```python
from build123d import *

# Parameters (mm, degrees)
BOSS_EXTRU_1_DEPTH      = 564
ESQUISSE2_W             = 18
ESQUISSE2_H             = 18
ENL_V_MAT_EXTRU_1_DEPTH = 3
ESQUISSE6_R             = 1.4
ENL_V_MAT_EXTRU_5_DEPTH = 3
SKETCH1_R               = 1.6
CUT_EXTRUDE1_DEPTH      = 21


with BuildPart() as part:
    # Esquisse1 → Boss.-Extru.1 (new body)
    with BuildSketch(Plane.XY):
        Polygon((0, 0), (20, 0), (20, 2), (2, 2), (2, 20), (0, 20), align=None)
    extrude(amount=BOSS_EXTRU_1_DEPTH)

    # Esquisse2 → Enlèv. mat.-Extru.1 (cut, through all)
    with BuildSketch(Plane(origin=(2, 0, 0), x_dir=(0, 0, -1), z_dir=(1, 0, 0))):
        with Locations((-555, 11)):
            Rectangle(ESQUISSE2_W, ESQUISSE2_H)
        with Locations((-9, 11)):
            Rectangle(ESQUISSE2_W, ESQUISSE2_H)
    extrude(amount=-ENL_V_MAT_EXTRU_1_DEPTH, mode=Mode.SUBTRACT)

    # Esquisse6 → Enlèv. mat.-Extru.5 (cut, through all)
    with BuildSketch(Plane(origin=(0, 2, 0), x_dir=(1, 0, 0), z_dir=(0, 1, 0))):
        with Locations((6.48, -549.52)):
            Circle(ESQUISSE6_R)
        with Locations((6.48, -14.48)):
            Circle(ESQUISSE6_R)
        with Locations((16.48, -559.52)):
            Circle(ESQUISSE6_R)
        with Locations((16.48, -4.48)):
            Circle(ESQUISSE6_R)
    extrude(amount=-ENL_V_MAT_EXTRU_5_DEPTH, mode=Mode.SUBTRACT)

    # Sketch1 → Cut-Extrude1 (cut, through all)
    with BuildSketch(Plane.ZY):
        with Locations((217, 11)):
            Circle(SKETCH1_R)
        with Locations((347, 11)):
            Circle(SKETCH1_R)
    extrude(amount=-CUT_EXTRUDE1_DEPTH, mode=Mode.SUBTRACT)


solid = part.part
```
Check sheet for the modelled part. Datum: model origin and axes. Units: mm. A direction names the side the tool comes from. Round coordinates to 2 decimals unless told otherwise and drop trailing zeros. Order: outer loops, then holes, each group sorted by start corner. A loop starts at its lowest first (then second) coordinate and runs counter-clockwise, first axis right, second up.
1) Scan lines: line 1 (Z direction, x = 16.48, y = 1.5); line 2 (Z direction, x = 6.48, y = 0.65); line 3 (X direction, y = 0.85, z = 549.52). Record each from-to range of solid material in increasing order.
2) Tool access check on faces 1 (the flat face through (2, 11, 278)), 2 (the flat face through (0, 10, 278)). Record the directions out of +Z, -Z, +X, -X, +Y, -Y that give a thin tool (end or side, any length) a straight path to the whole face; none if there is none.
3) Section check A-A (z = 431). Record the boundary of the cut face in (x, y).
4) Go/stop test with flat-tipped pins: pin 1 Ø4 at (y, z) = (11, 284.5) entering from +X; pin 2 Ø3 at (x, z) = (16.48, 559.52) entering from -Y; pin 3 Ø1 at (x, z) = (17, 382) entering from +Y; pin 4 Ø2 at (x, y) = (0.5, 11) entering from +Z. Record where each tip stops, or that it passes through.
5) Section check B-B (y = 6). Record the boundary of the cut face in (x, z), and give its area (3 significant figures).
Result:
1. line 1: z = 0 to 3.08, 5.88 to 558.12, 560.92 to 564
1. line 2: z = 0 to 13.08, 15.88 to 548.12, 550.92 to 564
1. line 3: x = 0 to 5.08, 7.88 to 20
2. face 1: +Z, -Z, +X, +Y
2. face 2: +Z, -Z, -X, +Y, -Y
3. outline: (0, 0) - (20, 0) - (20, 2) - (2, 2) - (2, 20) - (0, 20) - close
4. pin 1: stops at x = 2
4. pin 2: stops at y = 0
4. pin 3: stops at y = 2
4. pin 4: stops at z = 546
5. outline: (0, 18) - (2, 18) - (2, 546) - (0, 546) - close
5. area: 1,060 mm2
